from build123d import *

# Parameters (mm, degrees)
BOSS_EXTRUDE1_DEPTH = 5
SKETCH2_R           = 2.1
SKETCH2_R_2         = 2.5
SKETCH2_R_3         = 1.55
CUT_EXTRUDE1_DEPTH  = 151.602954818


with BuildPart() as part:
    # Sketch1 → Boss-Extrude1 (new body)
    with BuildSketch(Plane.XY):
        with BuildLine():
            Line((10.9658561, 6), (150, 6))
            Line((150, 6), (150, -6))
            Line((150, -6), (10.9658561, -6))
            ThreePointArc((10.9658561, -6), (-12.5, 0), (10.9658561, 6))
        make_face()
    extrude(amount=BOSS_EXTRUDE1_DEPTH)

    # Sketch2 → Cut-Extrude1 (cut, through all)
    with BuildSketch(Plane.XY.offset(5)):
        with Locations((140, 0)):
            Circle(SKETCH2_R)
        Circle(SKETCH2_R_2)
        with Locations((0, 8)):
            Circle(SKETCH2_R_3)
        with Locations((8, 0)):
            Circle(SKETCH2_R_3)
        with Locations((0, -8)):
            Circle(SKETCH2_R_3)
        with Locations((-8, 0)):
            Circle(SKETCH2_R_3)
    extrude(amount=-CUT_EXTRUDE1_DEPTH, mode=Mode.SUBTRACT)


solid = part.part
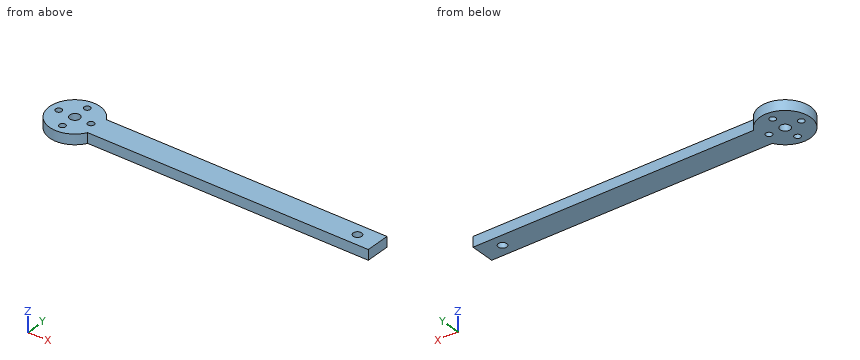
Read the model definition and answer for the solid it produces. Units are mm, in the model's axes. Coordinates: 2 decimals unless noted, no trailing zeros. Write each loop counter-clockwise with the first axis right and the second up, starting at its lowest first coordinate (ties: lowest second). Pieces come first, ordered by that corner, then holes. Notation, with made-up numbers: M 66,70 L 116,70 A12 cw 116,88 Z; hole C 58.25,84.25 d5. An arc over 180 degrees is marked long. Use a Markdown table: item, result.
Q1. Straight lines are drawn through the part: L1, parallel to Y at x = 0, z = 4.05; L2, parallel to X at y = -0.25, z = 3.45; L3, parallel to Y at x = 140, z = 1.8. For each, find the intervals that lie inside material, in ascending order. Write a range as [from, to].
Answer block:
| item | result |
|---|---|
| L1 | y = [-12.5, -9.55], [-6.45, -2.5], [2.5, 6.45], [9.55, 12.5] |
| L2 | x = [-12.5, -9.53], [-6.47, -2.49], [2.49, 6.47], [9.53, 137.91], [142.09, 150] |
| L3 | y = [-6, -2.1], [2.1, 6] |
Q2. The part is cut by section D-D, the plane x = 89. Write down the section's boundary in (y, z).
Answer block:
| item | result |
|---|---|
| outline | M -6,0 L 6,0 L 6,5 L -6,5 Z |
Q3. The part is cut by section C-C, the plane z = 3.75. Write down the section's boundary in (x, y), then the cut area to 3 significant figures.
Answer block:
| item | result |
|---|---|
| outline | M 10.97,-6 L 150,-6 L 150,6 L 10.97,6 A12.5 ccw long Z; hole C -8,0 d3.1; hole C 0,0 d5; hole C 0,-8 d3.1; hole C 0,8 d3.1; hole C 8,0 d3.1; hole C 140,0 d4.2 |
| area | 2,080 mm2 |
Q4. The part is cut by section A-A, the plane x = 140. Write down the section's boundary in (y, z).
Answer block:
| item | result |
|---|---|
| outline | M -6,0 L -2.1,0 L -2.1,5 L -6,5 Z; M 2.1,0 L 6,0 L 6,5 L 2.1,5 Z |
Q5. The part is cut by section B-B, the plane y = -8. Write down the section's boundary in (x, z).
Answer block:
| item | result |
|---|---|
| outline | M -9.6,0 L -1.55,0 L -1.55,5 L -9.6,5 Z; M 1.55,0 L 9.6,0 L 9.6,5 L 1.55,5 Z |
Q6. Each of these flat-tipped pins is pushed along its axis until it touches: pin 1 Ø6 at (x, y) = (26.5, -1.5) entering from -Z; pin 2 Ø2.5 at (x, z) = (99, 1.5) entering from +Y. Where does it stop, or does it pass through?
Answer block:
| item | result |
|---|---|
| pin 1 | stops at z = 0 |
| pin 2 | stops at y = 6 |
